from build123d import *

# Parameters (mm, degrees)
EXTRUDE_1_DEPTH          = 163
EXTRUDE_2_DEPTH          = 2
EXTRUDE_3_DEPTH          = 2
SKETCH_4_W               = 37
SKETCH_4_H               = 10
EXTRUDE_4_DEPTH          = 2
SKETCH_5_W               = 71.5
SKETCH_5_H               = 24.5
CUT_EXTRUDE_1_DEPTH      = 186.248481775
SKETCH_6_W               = 79.5
SKETCH_6_H               = 32.5
SKETCH_6_W_2             = 71.5
SKETCH_6_H_2             = 24.5
EXTRUDE_5_DEPTH          = 3
EXTRUDE_6_DEPTH          = 79.5
SKETCH_10_R              = 15
CUT_EXTRUDE_2_DEPTH      = 14
EXTRUDE_8_DEPTH          = 14
SKETCH_12_R              = 3.75
EXTRUDE_9_DEPTH          = 3
CUT_EXTRUDE_3_DEPTH      = 186.137402806
CUT_EXTRUDE_3_DEPTH_BACK = 186.137402806
SKETCH_14_W              = 17.5
SKETCH_14_H              = 13
SKETCH_15_W              = 23.5
SKETCH_15_H              = 19
SKETCH_15_W_2            = 17.5
SKETCH_15_H_2            = 13
EXTRUDE_10_DEPTH         = 0.5
SKETCH_16_W              = 23.5
SKETCH_16_H              = 19
EXTRUDE_11_DEPTH         = 2
CHAMFER_2_SIZE           = 2
CHAMFER_3_SIZE           = 1.5
SKETCH_17_R              = 0.85
CUT_EXTRUDE_4_DEPTH      = 10
SKETCH_18_W              = 5
SKETCH_18_H              = 7
EXTRUDE_12_DEPTH         = 161
SKETCH_19_R              = 2.1
CUT_EXTRUDE_5_DEPTH      = 161
SKETCH_20_W              = 5
SKETCH_20_H              = 8
EXTRUDE_13_DEPTH         = 22
SKETCH_21_R              = 2.1
CUT_EXTRUDE_6_DEPTH      = 30.1
EXTRUDE_14_DEPTH         = 161
CUT_EXTRUDE_7_DEPTH      = 185.983783073
CUT_EXTRUDE_7_DEPTH_BACK = 185.983783073
SKETCH_23_R              = 2.1
EXTRUDE_15_DEPTH         = 2
EXTRUDE_16_DEPTH         = 6
FILLET_1_R               = 6
CHAMFER_5_SIZE           = 3
CHAMFER_5_SIZE2          = 5.196152423


with BuildPart() as part:
    # Эскиз1 → Бобышка-Вытянуть1 (new body)
    with BuildSketch(Plane.XY):
        Polygon((0, 0), (-31, 31), (-81, 31), (-81, 33), (-31, 33), (2, 0), align=None)
    extrude(amount=EXTRUDE_1_DEPTH)

    # Эскиз2 → Бобышка-Вытянуть2 (add)
    with BuildSketch(Plane.XY.offset(163)):
        Polygon((2, 0), (-31, 33), (-79, 33), (-79, 0), align=None)
    extrude(amount=-EXTRUDE_2_DEPTH)

    # Эскиз3 → Бобышка-Вытянуть3 (add)
    with BuildSketch(Plane(origin=(0, 0, 0), x_dir=(-1, 0, 0), z_dir=(0, 0, -1))):
        Polygon((0, 0), (31, 31), (79, 31), (79, 28), (32.242640687, 28), (4.242640687, 0), align=None)
    extrude(amount=-EXTRUDE_3_DEPTH)

    # Эскиз4 → Бобышка-Вытянуть4 (add)
    with BuildSketch(Plane.XZ):
        with Locations((-60.5, 156)):
            Rectangle(SKETCH_4_W, SKETCH_4_H)
    extrude(amount=-EXTRUDE_4_DEPTH)

    # Эскиз5 → Вырез-Вытянуть1 (cut, through all)
    with BuildSketch(Plane(origin=(1, 1, 0), x_dir=(0, 0, -1), z_dir=(0.7071067811865461, 0.7071067811865489, 0))):
        with Locations((-77.25, 23.840620434)):
            Rectangle(SKETCH_5_W, SKETCH_5_H)
    extrude(amount=-CUT_EXTRUDE_1_DEPTH, mode=Mode.SUBTRACT)

    # Эскиз6 → Бобышка-Вытянуть5 (add)
    with BuildSketch(Plane(origin=(0, 0, 0), x_dir=(0, 0, 1), z_dir=(-0.7071067811865462, -0.7071067811865489, 0))):
        with Locations((77.25, 23.840620434)):
            Rectangle(SKETCH_6_W, SKETCH_6_H)
        with Locations((77.25, 23.840620434)):
            Rectangle(SKETCH_6_W_2, SKETCH_6_H_2, mode=Mode.SUBTRACT)
    extrude(amount=EXTRUDE_5_DEPTH)

    # Эскиз8 → Бобышка-Вытянуть6 (add)
    with BuildSketch(Plane(origin=(0, 0, 37.5), x_dir=(-1, 0, 0), z_dir=(0, 0, -1))):
        Polygon((28.348349571, 28.348349571), (30.469669914, 26.227029227), (35.242640687, 31), (31, 31), align=None)
    extrude(amount=-EXTRUDE_6_DEPTH)

    # Эскиз10 → Вырез-Вытянуть2 (cut)
    with BuildSketch(Plane(origin=(1, 1, 0), x_dir=(0, 0, -1), z_dir=(0.7071067811865461, 0.7071067811865489, 0))):
        with Locations((-150, 25.254833996)):
            Circle(SKETCH_10_R)
    extrude(amount=-CUT_EXTRUDE_2_DEPTH, mode=Mode.SUBTRACT)

    # Эскиз11 → Бобышка-Вытянуть8 (add)
    with BuildSketch(Plane(origin=(1, 1, 0), x_dir=(0, 0, -1), z_dir=(0.7071067811865461, 0.7071067811865489, 0))):
        with BuildLine():
            Line((-163, 32.738148769), (-163, 35.738148769))
            ThreePointArc((-163, 35.738148769), (-133.299703936, 25.254833996), (-163, 14.771519222))
            Line((-163, 14.771519222), (-163, 17.771519222))
            ThreePointArc((-163, 17.771519222), (-135, 25.254833996), (-163, 32.738148769))
        make_face()
    extrude(amount=-EXTRUDE_8_DEPTH)

    # Эскиз12 → Бобышка-Вытянуть9 (add)
    with BuildSketch(Plane(origin=(-8.899494937, -8.899494937, 0), x_dir=(0, 0, -1), z_dir=(0.7071067811865461, 0.7071067811865489, 0))):
        with BuildLine():
            Line((-163, 35.737677122), (-163, 14.77199087))
            ThreePointArc((-163, 14.77199087), (-133.3, 25.254833996), (-163, 35.737677122))
        make_face()
        with Locations(Location((-150, 25.254833996, 0), (0, 0, 270))):
            Circle(SKETCH_12_R, mode=Mode.SUBTRACT)
    extrude(amount=EXTRUDE_9_DEPTH)

    # Эскиз14 → Вырез-Вытянуть3 (cut, two sides: drawn at the far end of the back side and taken through both)
    with BuildSketch(Plane.XZ.offset(-31).offset(-CUT_EXTRUDE_3_DEPTH_BACK)):
        with Locations((-49.75, 23.5)):
            Rectangle(SKETCH_14_W, SKETCH_14_H)
    extrude(amount=CUT_EXTRUDE_3_DEPTH + CUT_EXTRUDE_3_DEPTH_BACK, mode=Mode.SUBTRACT)

    # Эскиз15 → Бобышка-Вытянуть10 (add)
    with BuildSketch(Plane.XZ.offset(-31)):
        with Locations((-49.75, 23.5)):
            Rectangle(SKETCH_15_W, SKETCH_15_H)
        with Locations((-49.75, 23.5)):
            Rectangle(SKETCH_15_W_2, SKETCH_15_H_2, mode=Mode.SUBTRACT)
    extrude(amount=EXTRUDE_10_DEPTH)

    # Эскиз16 → Бобышка-Вытянуть11 (add)
    with BuildSketch(Plane.XZ.offset(-30.5)):
        with Locations((-49.75, 23.5)):
            Rectangle(SKETCH_16_W, SKETCH_16_H)
    extrude(amount=EXTRUDE_11_DEPTH)

    # Фаска2
    chamfer_2_edges = [part.edges().sort_by_distance(p)[0] for p in [
        (-38, 31, 23.5),
        (-49.75, 31, 33),
        (-61.5, 31, 23.5),
        (-49.75, 31, 14),
    ]]
    chamfer(chamfer_2_edges, length=CHAMFER_2_SIZE)

    # Фаска3
    chamfer_3_edges = [part.edges().sort_by_distance(p)[0] for p in [
        (-41, 33, 23.5),
        (-49.75, 33, 17),
        (-58.5, 33, 23.5),
        (-49.75, 33, 30),
    ]]
    chamfer(chamfer_3_edges, length=CHAMFER_3_SIZE)

    # Эскиз17 → Вырез-Вытянуть4 (cut)
    with BuildSketch(Plane(origin=(0, 30.5, 0), x_dir=(1, 0, 0), z_dir=(0, 1, 0))):
        with Locations(Location((-57.65, -20, 0), (0, 0, 270))):
            Circle(SKETCH_17_R)
        with Locations(Location((-57.65, -22.54, 0), (0, 0, 270))):
            Circle(SKETCH_17_R)
        with Locations(Location((-57.65, -25.08, 0), (0, 0, 270))):
            Circle(SKETCH_17_R)
        with Locations(Location((-57.65, -27.62, 0), (0, 0, 270))):
            Circle(SKETCH_17_R)
    extrude(amount=-CUT_EXTRUDE_4_DEPTH, mode=Mode.SUBTRACT)

    # Эскиз18 → Бобышка-Вытянуть12 (add)
    with BuildSketch(Plane(origin=(0, 0, 161), x_dir=(-1, 0, 0), z_dir=(0, 0, -1))):
        with Locations((76.5, 27.5)):
            Rectangle(SKETCH_18_W, SKETCH_18_H)
    extrude(amount=EXTRUDE_12_DEPTH)

    # Эскиз19 → Вырез-Вытянуть5 (cut)
    with BuildSketch(Plane(origin=(0, 0, 0), x_dir=(-1, 0, 0), z_dir=(0, 0, -1))):
        with Locations((79, 28)):
            Circle(SKETCH_19_R)
    extrude(amount=-CUT_EXTRUDE_5_DEPTH, mode=Mode.SUBTRACT)

    # Эскиз20 → Бобышка-Вытянуть13 (add)
    with BuildSketch(Plane.XZ.offset(-24)):
        with Locations((-76.5, 157)):
            Rectangle(SKETCH_20_W, SKETCH_20_H)
    extrude(amount=EXTRUDE_13_DEPTH)

    # Эскиз21 → Вырез-Вытянуть6 (cut)
    with BuildSketch(Plane.XZ):
        with Locations((-79, 159)):
            Circle(SKETCH_21_R)
    extrude(amount=-CUT_EXTRUDE_6_DEPTH, mode=Mode.SUBTRACT)

    # Эскиз22 → Бобышка-Вытянуть14 (add)
    with BuildSketch(Plane(origin=(0, 0, 161), x_dir=(-1, 0, 0), z_dir=(0, 0, -1))):
        Polygon((4.5, -1.5), (4.5, 4.5), (0, 0), (0, -6.5), (4.5, -6.5), align=None)
    extrude(amount=EXTRUDE_14_DEPTH)

    # Эскиз23 → Вырез-Вытянуть7 (cut, two sides: drawn at the far end of the back side and taken through both)
    with BuildSketch(Plane(origin=(0, 0, 0), x_dir=(-1, 0, 0), z_dir=(0, 0, -1)).offset(-CUT_EXTRUDE_7_DEPTH_BACK)):
        with Locations((0, -3)):
            Circle(SKETCH_23_R)
    extrude(amount=CUT_EXTRUDE_7_DEPTH + CUT_EXTRUDE_7_DEPTH_BACK, mode=Mode.SUBTRACT)

    # Эскиз24 → Бобышка-Вытянуть15 (add)
    with BuildSketch(Plane(origin=(0, 0, 0), x_dir=(-1, 0, 0), z_dir=(0, 0, -1))):
        Polygon((74, 24), (74, 28), (32.242640687, 28), (4.5, 0.257359313), (4.5, -3.742640687), (32.242640687, 24), align=None)
    extrude(amount=-EXTRUDE_15_DEPTH)

    # Эскиз25 → Бобышка-Вытянуть16 (add)
    with BuildSketch(Plane(origin=(0, 2, 0), x_dir=(1, 0, 0), z_dir=(0, 1, 0))):
        Polygon((-42, -151), (-79, -151), (-79, -149), (-40, -149), (-40, -159), (-4.5, -159), (-4.5, -161), (-42, -161), align=None)
    extrude(amount=-EXTRUDE_16_DEPTH)

    # Скругление1
    fillet_1_edges = [part.edges().sort_by_distance(p)[0] for p in [
        (-40, -1, 149),
    ]]
    fillet(fillet_1_edges, radius=FILLET_1_R)

    # Фаска5
    chamfer_5_edges = [part.edges().sort_by_distance(p)[0] for p in [
        (-46.899494937, 2, 161),
    ]]
    chamfer_5_side = [part.faces().sort_by_distance(p)[0] for p in [
        (-55.732444542, 2, 155.342995901),
    ]]
    chamfer(chamfer_5_edges, length=CHAMFER_5_SIZE, length2=CHAMFER_5_SIZE2, reference=chamfer_5_side[0])


solid = part.part
Verification items for the finished model (mm, model axes). A direction names the side the tool comes from. Give positions to 0.01 mm unless a question says otherwise; leave off trailing zeros. Order: outer loops, then holes, each group sorted by start corner. A loop starts at its lowest first (then second) coordinate and runs counter-clockwise, first axis right, second up. Notation, with made-up numbers: M -39,50.5 L -11,50.5 A28 cw -11,87.5 Z; hole C 25.5,86.5 d10. An arc over 180 degrees is marked long. Answer as a JSON object with one key per item and string values. Group by question number.
1) Cross-section at A-A (z = 103). Enter the section's corners in (x, y).
2) Depth check by flat-ended pin: pin 1 Ø1.5 at (x, y) = (-76.5, 18.5) entering from -Z; pin 2 Ø1.5 at (x, z) = (-17, 141) entering from +Y; pin 3 Ø4 at (x, z) = (-14, 23.5) entering from -Y; pin 4 Ø1.4 at (x, z) = (-57.65, 22.54) entering from +Y. Enter the tip coordinate at first touch or a pass-through.
3) Scan lines: line 1 along Y through (x, z) = (-62, 151.5); line 2 along Y through (x, z) = (-75, 151.5); line 3 along Z through (x, y) = (-9.5, 6.5). Record each from-to range of solid material in increasing order. Write a range as [from, to].
4) Cross-section at B-B (x = -72). Enter the section's corners in (y, z), then the cut area to 3 significant figures.
5) Mould release check, pull along X, two halves, no side actions. Record for faces 5 (the face through (-20, 17, 37.5)), 6 (the face through (0.3, 0, 118.1)), 7 (the face through (-4, 6, 80)), 8 (the face through (-79, 30.5, 81.1)): released by +X, released by -X, zero draft, split by the parting line, or undercut.
6) Access from +Z, -Z, +X, -X, +Y, -Y to the whole of each face (thin tool, end or side, straight path). Record for faces 1 (the face through (-74, 26, 87)), 2 (the face through (-8.73, 7.66, 76.75)), 3 (the face through (-60, -2, 151)), 4 (the face through (-21, -2, 161)).
Result sheet:
{
 "1": {"outline": "M -81,31 L -79,31 L -79,30.1 A2.1 cw -79,25.9 L -79,24 L -74,24 L -74,31 L -35.24,31 L -27.64,23.4 L -24.52,26.52 L -31,33 L -81,33 Z; M -10.32,6.07 L -7.49,3.25 L -5.37,5.37 L -4.5,4.5 L -4.5,-6.5 L 0,-6.5 L 0,-5.1 A2.1 cw 0,-0.9 L 0,0 L 2,0 L -7.2,9.2 Z"},
 "2": {"pin 1": "stops at z = 153", "pin 2": "stops at y = 4.19", "pin 3": "stops at y = 12", "pin 4": "passes through"},
 "3": {"line 1": "y = [0, 2], [31, 33]", "line 2": "y = [0, 2], [24, 33]", "line 3": "z = [0, 2], [37.5, 117], [140.81, 144.46], [155.54, 159.19], [161, 163]"},
 "4": {"outline": "M -4,149 L 2,149 L 2,158 L 7.2,161 L 31,161 L 31,2 L 24,2 L 24,0 L 33,0 L 33,163 L 0,163 L 0,151 L -4,151 Z", "area": "442 mm2"},
 "5": {"face 5": "undercut", "face 6": "zero draft", "face 7": "released by +X", "face 8": "released by -X"},
 "6": {"face 1": "none", "face 2": "-X, +Y", "face 3": "+Z, -X, -Y", "face 4": "+Z, +X, -X, -Y"}
}
